Source: CAD feature listing. Evaluate the final solid. Frame: model axes, mm. Give positions to 0.01 mm unless a question says otherwise; leave off trailing zeros. Order: outer loops, then holes, each group sorted by start corner. A loop starts at its lowest first (then second) coordinate and runs counter-clockwise, first axis right, second up. Notation, with made-up numbers: (62, 8.25) - (116, 8.25) arc R32 cw to (116, 46.25) - close; hole circle Ø4 at (71, 43). An arc over 180 degrees is marked (long way). One line per item, written item: value. Start each with the question number.
from build123d import *

# Parameters (mm, degrees)
SKETCH_R    = 3
PAD_DEPTH   = 10
FILLET_R    = 20
FILLET001_R = 1.6
FILLET002_R = 1


with BuildPart() as part:
    # Sketch → Pad (new body)
    with BuildSketch(Plane.XY):
        with BuildLine():
            ThreePointArc((-36.66369, 93.5), (-24, 100), (-36.66369, 106.5))
            Line((-46, 106.5), (-36.66369, 106.5))
            Line((-46, 106.5), (-46, 104))
            Line((-46, 104), (-72, 104))
            Line((-72, 159.5), (-72, 104))
            Line((53, 159.5), (-72, 159.5))
            Line((53, 40.5), (53, 159.5))
            Line((-72, 40.5), (53, 40.5))
            Line((-72, 96), (-72, 40.5))
            Line((-46, 96), (-72, 96))
            Line((-46, 93.5), (-46, 96))
            Line((-46, 93.5), (-36.66369, 93.5))
        make_face()
        with Locations((-57, 133)):
            Circle(SKETCH_R, mode=Mode.SUBTRACT)
        with Locations((-57, 67)):
            Circle(SKETCH_R, mode=Mode.SUBTRACT)
        with Locations((38, 133)):
            Circle(SKETCH_R, mode=Mode.SUBTRACT)
        with Locations((38, 67)):
            Circle(SKETCH_R, mode=Mode.SUBTRACT)
        with BuildLine():
            ThreePointArc((-4.5, 152.5), (-7.5, 149.5), (-4.5, 146.5))
            Line((-4.5, 146.5), (30.5, 146.5))
            ThreePointArc((30.5, 146.5), (33.5, 149.5), (30.5, 152.5))
            Line((-4.5, 152.5), (30.5, 152.5))
        make_face(mode=Mode.SUBTRACT)
        with BuildLine():
            ThreePointArc((-4.5, 119.5), (-7.5, 116.5), (-4.5, 113.5))
            Line((-4.5, 113.5), (30.5, 113.5))
            ThreePointArc((30.5, 113.5), (33.5, 116.5), (30.5, 119.5))
            Line((-4.5, 119.5), (30.5, 119.5))
        make_face(mode=Mode.SUBTRACT)
        with BuildLine():
            ThreePointArc((-4.5, 86.5), (-7.5, 83.5), (-4.5, 80.5))
            Line((-4.5, 80.5), (30.5, 80.5))
            ThreePointArc((30.5, 80.5), (33.5, 83.5), (30.5, 86.5))
            Line((-4.5, 86.5), (30.5, 86.5))
        make_face(mode=Mode.SUBTRACT)
        with BuildLine():
            ThreePointArc((-4.5, 53.5), (-7.5, 50.5), (-4.5, 47.5))
            Line((-4.5, 47.5), (30.5, 47.5))
            ThreePointArc((30.5, 47.5), (33.5, 50.5), (30.5, 53.5))
            Line((-4.5, 53.5), (30.5, 53.5))
        make_face(mode=Mode.SUBTRACT)
    extrude(amount=PAD_DEPTH)

    # Fillet
    fillet_edges = [part.edges().sort_by_distance(p)[0] for p in [
        (-72, 159.5, 5),
        (53, 40.5, 5),
        (-72, 40.5, 5),
        (53, 159.5, 5),
    ]]
    fillet(fillet_edges, radius=FILLET_R)

    # Fillet001
    fillet001_edges = [part.edges().sort_by_distance(p)[0] for p in [
        (-46, 106.5, 5),
        (-46, 93.5, 5),
    ]]
    fillet(fillet001_edges, radius=FILLET001_R)

    # Fillet002
    fillet002_edges = [part.edges().sort_by_distance(p)[0] for p in [
        (-72, 104, 5),
        (-72, 96, 5),
    ]]
    fillet(fillet002_edges, radius=FILLET002_R)


solid = part.part
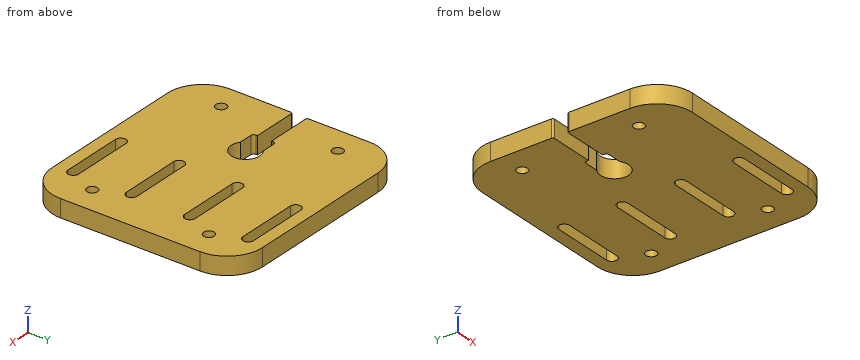
1. Section D-D on y = 67. Return the cut outline in (x, z), then the cut area to 3 significant figures.
2. Section B-B on x = -2. Return the cut outline in (y, z).
3. Section A-A on y = 83.5. Return the cut outline in (x, z).
4. Section C-C on x = -57. Return the cut outline in (y, z).
5. Contact query for flat-ended pins moving along their axis: pin 1 Ø7 at (x, y) = (-57, 133) entering from +Z; pin 2 Ø5 at (x, z) = (-62, 4.5) entering from -Y; pin 3 Ø1 at (x, z) = (-53, 1.5) entering from -Y; pin 4 Ø3 at (x, z) = (38, 1) entering from -Y. Output: stop coordinate, or through.
6. Ray query, L1, parallel to X at y = 133, z = 7.75; L2, parallel to Y at x = 1.5, z = 4.25; L3, parallel to Y at x = -32, z = 8.25. Return the intervals inside material, ascending.
Data:
1. outline: (-72, 0) - (-60, 0) - (-60, 10) - (-72, 10) - close; (-54, 0) - (35, 0) - (35, 10) - (-54, 10) - close; (41, 0) - (53, 0) - (53, 10) - (41, 10) - close
1. area: 1,130 mm2
2. outline: (40.5, 0) - (47.5, 0) - (47.5, 10) - (40.5, 10) - close; (53.5, 0) - (80.5, 0) - (80.5, 10) - (53.5, 10) - close; (86.5, 0) - (113.5, 0) - (113.5, 10) - (86.5, 10) - close; (119.5, 0) - (146.5, 0) - (146.5, 10) - (119.5, 10) - close; (152.5, 0) - (159.5, 0) - (159.5, 10) - (152.5, 10) - close
3. outline: (-72, 0) - (-7.5, 0) - (-7.5, 10) - (-72, 10) - close; (33.5, 0) - (53, 0) - (53, 10) - (33.5, 10) - close
4. outline: (41.14, 0) - (64, 0) - (64, 10) - (41.14, 10) - close; (70, 0) - (96, 0) - (96, 10) - (70, 10) - close; (104, 0) - (130, 0) - (130, 10) - (104, 10) - close; (136, 0) - (158.86, 0) - (158.86, 10) - (136, 10) - close
5. pin 1: stops at z = 10
5. pin 2: stops at y = 41.96
5. pin 3: stops at y = 40.51
5. pin 4: stops at y = 40.81
6. L1: x = -72 to -60, -54 to 35, 41 to 53
6. L2: y = 40.5 to 47.5, 53.5 to 80.5, 86.5 to 113.5, 119.5 to 146.5, 152.5 to 159.5
6. L3: y = 40.5 to 92, 108 to 159.5
